Design review of the part built by this model. Coordinates are the model's own, in mm. A direction names the side the tool comes from. Coordinates: 2 decimals unless noted, no trailing zeros. Order: outer loops, then holes, each group sorted by start corner. A loop starts at its lowest first (then second) coordinate and runs counter-clockwise, first axis right, second up. Notation, with made-up numbers: M 19,-37 L 47,-37 A20 ccw 47,-12 Z; hole C 66,14 d11. An arc over 180 degrees is marked long. Answer as a JSON object with one key per item and string values.
from build123d import *

# Parameters (mm, degrees)
SKETCH005_W     = 102.620446
SKETCH005_H     = 81.982758
PAD005_DEPTH    = 3
SKETCH006_W     = 102.620446
SKETCH006_H     = 81.982758
SKETCH006_W_2   = 40
SKETCH006_H_2   = 20
PAD006_DEPTH    = 1
PAD006_FACE18_W = 20
PAD006_FACE18_H = 40
POCKET_DEPTH    = 3.001
SKETCH007_R     = 31
SKETCH007_R_2   = 29.055
PAD007_DEPTH    = 3
PAD013_DEPTH    = 6
SKETCH014_W     = 40
SKETCH014_H     = 20
PAD014_DEPTH    = 3


with BuildPart() as part:
    # Sketch005 → Pad005 (new body)
    with BuildSketch(Plane.XY):
        Rectangle(SKETCH005_W, SKETCH005_H)
        with BuildLine():
            ThreePointArc((-21.953744, 12.675), (0, -25.35), (21.953744, 12.675))
            ThreePointArc((-21.953744, 12.675), (0, -28.406865), (21.953744, 12.675))
        make_face(mode=Mode.SUBTRACT)
    extrude(amount=PAD005_DEPTH)

    # Sketch006 (on Face8 of Pad005) → Pad006 (join)
    with BuildSketch(Plane.XY.offset(3)):
        Rectangle(SKETCH006_W, SKETCH006_H)
        Rectangle(SKETCH006_W_2, SKETCH006_H_2, mode=Mode.SUBTRACT)
    extrude(amount=PAD006_DEPTH)

    # Pad006 Face18 → Pocket (cut, through all)
    with BuildSketch(Plane(origin=(0, 0, 3), x_dir=(0, 1, 0), z_dir=(0, 0, 1))):
        Rectangle(PAD006_FACE18_W, PAD006_FACE18_H)
    extrude(amount=-POCKET_DEPTH, mode=Mode.SUBTRACT)

    # Sketch007 (on Face4 of Pocket) → Pad007 (join)
    with BuildSketch(Plane(origin=(0, 0, 0), x_dir=(1, 0, 0), z_dir=(0, 0, -1))):
        with Locations((0, 2)):
            Circle(SKETCH007_R)
        with Locations((0, 2)):
            Circle(SKETCH007_R_2, mode=Mode.SUBTRACT)
    extrude(amount=PAD007_DEPTH)

    # Sketch013 (on Face10 of Pad007) → Pad013 (join)
    with BuildSketch(Plane.XY.offset(4)):
        with BuildLine():
            Line((51.310223, 25), (51.310223, 15))
            Line((51.310223, 15), (-20, 15))
            Line((-20, 15), (-20, -18))
            Line((-20, -18), (21, -18))
            ThreePointArc((25, -22), (23.828427, -19.171573), (21, -18))
            Line((25, -22), (25, -23))
            Line((25, -23), (-30, -23))
            Line((-30, -23), (-30, 25))
            Line((-30, 25), (51.310223, 25))
        make_face()
    extrude(amount=PAD013_DEPTH)

    # Sketch014 (on Face25 of Pad013) → Pad014 (join)
    with BuildSketch(Plane.XY.offset(10)):
        Polygon((51.310223, 25), (25, -23), (-30, -23), (-30, 25), align=None)
        Rectangle(SKETCH014_W, SKETCH014_H, mode=Mode.SUBTRACT)
    extrude(amount=PAD014_DEPTH)


with BuildPart() as part_1:
    # Body002 placement: moved
    add(part.part.moved(Location((0, 0, 30))))


solid = part_1.part
1) Add section D-D (z = 37.25). State the section outline as (x, y) points.
Taken from the geometry:
{"outline": "M -30,-23 L 25,-23 L 25,-22 A4 ccw 21,-18 L -20,-18 L -20,15 L 51.31,15 L 51.31,25 L -30,25 Z"}
2) Add section C-C (z = 31.25). State the section outline as (x, y) points (3 decimals), and give its area (3 significant figures).
Taken from the geometry:
{"outline": "M -51.31,-40.991 L 51.31,-40.991 L 51.31,40.991 L -51.31,40.991 Z; hole M -21.954,12.675 A26.407 ccw long 21.954,12.675 A25.35 cw long Z; hole M -20,-10 L 20,-10 L 20,10 L -20,10 Z", "area": "7,410 mm2"}
3) Add section B-B (y = -2). Count the separate pieces of the cut face and the enclosed holes in it, and give its area (3 significant figures).
Taken from the geometry:
{"separate pieces": "3", "enclosed holes": "0", "area": "395 mm2"}
4) Mouldability with a two-part tool opening along Z and no side actions: class faces 6 (the cylindrical face through (23.859, -19.203, 36.958)), 7 (the flat face through (0, -26, 33)), 8 (the cylindrical face through (-3.78, -30.81, 28.52)) as released by +Z, released by -Z, zero draft, split by the parting line, or undercut.
Taken from the geometry:
{"face 6": "undercut", "face 7": "released by -Z", "face 8": "zero draft"}
5) Tool access review of faces 1 (the cylindrical face through (-4.036, -32.736, 28.521)), 2 (the flat face through (-20, -1, 36)), 3 (the flat face through (16, 15, 37)), 4 (the flat face through (50, 18, 40)), 5 (the flat face through (20, 0, 32)): name each direction out of +Z, -Z, +X, -X, +Y, -Y from which nothing blocks a thin tool from reaching the whole face with its end or side.
Taken from the geometry:
{"face 1": "-Z", "face 2": "none", "face 3": "+X", "face 4": "+Z, +X, -Y", "face 5": "+Z, -Z"}
6) Insertion check: pin 1 Ø17.5 at (x, y) = (-13.5, -9.5) entering from -Z; pin 2 Ø3 at (x, z) = (29.5, 38) entering from -Y; pin 3 Ø1.8 at (x, z) = (-6, 36) entering from +Y. Each pin has a flat end and moves straight along its axis. Give the tip position at first contact, or say it passes through.
Taken from the geometry:
{"pin 1": "stops at z = 30", "pin 2": "stops at y = 15", "pin 3": "stops at y = 25"}
7) To check wall thickness, follow L1, parallel to Z at x = 25, y = -5.5; L2, parallel to Y at x = 0, z = 28.3 (3 decimals); L3, parallel to Z at x = 18, y = -29.5. State the ranges of each line that lie inside material, in increasing order.
Taken from the geometry:
{"L1": "z = 33 to 34, 40 to 43", "L2": "y = -33 to -31.055, 27.055 to 29", "L3": "z = 30 to 34"}
